Can you work these out from the model? Positions are in its coordinate system, mm. A direction names the side the tool comes from. Coordinates: 2 decimals unless noted, no trailing zeros. Loops run counter-clockwise (first coordinate to the right, second up) from the corner with the lowest first, then second, coordinate; pieces in that order, holes last.
```python
from build123d import *

# Parameters (mm, degrees)
SKETCH_W        = 16.8
SKETCH_H        = 16.8
SKETCH_R        = 2
PAD_DEPTH       = 16
SKETCH002_R     = 2
SKETCH002_R_2   = 3
PAD001_DEPTH    = 4
SKETCH003_W     = 12.4
SKETCH003_H     = 11.9
POCKET001_DEPTH = 12
SKETCH001_R     = 3.5
POCKET_DEPTH    = 4
POCKET002_DEPTH = 3.5
SKETCH005_R     = 2
POCKET003_DEPTH = 38.401
FILLET_R        = 2


with BuildPart() as part:
    # Sketch → Pad (new body)
    with BuildSketch(Plane.XY):
        Rectangle(SKETCH_W, SKETCH_H)
        Circle(SKETCH_R, mode=Mode.SUBTRACT)
    extrude(amount=PAD_DEPTH)

    # Sketch002 → Pad001 (join)
    with BuildSketch(Plane.XY.offset(16)):
        Polygon((-10, -10), (30, -10), (30, 10), (10, 10), (10, 30), (-10, 30), align=None)
        Circle(SKETCH002_R, mode=Mode.SUBTRACT)
        with Locations((0, 13.25)):
            Circle(SKETCH002_R_2, mode=Mode.SUBTRACT)
        with Locations((13.25, 0)):
            Circle(SKETCH002_R_2, mode=Mode.SUBTRACT)
    extrude(amount=PAD001_DEPTH)

    # Sketch003 → Pocket001 (cut)
    with BuildSketch(Plane.XY):
        with Locations((2.2, 2.45)):
            Rectangle(SKETCH003_W, SKETCH003_H)
    extrude(amount=POCKET001_DEPTH, mode=Mode.SUBTRACT)

    # Sketch001 (on Face5 of Pocket001) → Pocket (cut)
    with BuildSketch(Plane(origin=(0, 0, 16), x_dir=(1, 0, 0), z_dir=(0, 0, -1))):
        Circle(SKETCH001_R)
    extrude(amount=POCKET_DEPTH, mode=Mode.SUBTRACT)

    # Sketch004 (on Face7 of Pocket) → Pocket002 (cut)
    with BuildSketch(Plane(origin=(0, -3.5, 0), x_dir=(-1, 0, 0), z_dir=(0, 1, 0))):
        Polygon((4, 6), (2, 9.464102), (-2, 9.464102), (-4, 6), (-2, 2.535898), (2, 2.535898), align=None)
    extrude(amount=-POCKET002_DEPTH, mode=Mode.SUBTRACT)

    # Sketch005 (on Face1 of Pocket002) → Pocket003 (cut, through all)
    with BuildSketch(Plane.XZ.offset(8.4)):
        with Locations((0, 6)):
            Circle(SKETCH005_R)
    extrude(amount=-POCKET003_DEPTH, mode=Mode.SUBTRACT)

    # Fillet
    fillet_edges = [part.edges().sort_by_distance(p)[0] for p in [
        (-10, 30, 18),
        (10, 30, 18),
        (30, 10, 18),
        (30, -10, 18),
    ]]
    fillet(fillet_edges, radius=FILLET_R)


solid = part.part
```
Item 1: Suppose I cut it at A-A, the plane y = 13.25. Please give me the cut outline in (x, z).
Results are:
outline: (-10, 16) - (-3, 16) - (-3, 20) - (-10, 20) - close; (3, 16) - (10, 16) - (10, 20) - (3, 20) - close
Item 2: I need wall thicknesses on line 1 along Y through (x, z) = (0, 18.3); line 2 along Y through (x, z) = (13.25, 18.25); line 3 along X through (y, z) = (0, 15.15). Which ranges of each line are inside material? Lowest first, please.
Results are:
line 1: y = -10 to -2, 2 to 10.25, 16.25 to 30
line 2: y = -10 to -3, 3 to 10
line 3: x = -8.4 to -3.5, 3.5 to 8.4
Item 3: Suppose I cut it at D-D, the plane z = 5.25. Please give me the cut outline in (x, y).
Results are:
outline: (-8.4, -8.4) - (-1.85, -8.4) - (-1.85, -7) - (-3.57, -7) - (-3.57, -3.5) - (-4, -3.5) - (-4, 8.4) - (-8.4, 8.4) - close; (1.85, -8.4) - (8.4, -8.4) - (8.4, -3.5) - (3.57, -3.5) - (3.57, -7) - (1.85, -7) - close
Item 4: On a 3-axis mill with a long thin cutter (end or side, diameter ignored), from which of +Z, -Z, +X, -X, +Y, -Y can I reach the whole of each face in a straight line? I mean faces 1 (the face through (0, -8.4, 10)), 2 (the face through (-3.014, -5.226, 7.708)), 3 (the face through (19, 10, 18)), 4 (the face through (9, -10, 18)), 5 (the face through (-4, 8.4, 13)). Say none if no direction works.
Results are:
face 1: -Z, +X, -X, -Y
face 2: +Y
face 3: +Z, -Z, +X, +Y
face 4: +Z, -Z, +X, -X, -Y
face 5: -Z, +X, -X, +Y
Item 5: I'm going to push flat-ended pins straight in: P1, Ø6, axis at y = 21, z = 14, coming from the +X side; P2, Ø3.5, axis at x = 0.5, z = 7.5, coming from the +Y side; P3, Ø1, axis at y = -1, z = 5.5, coming from the +X side. Where does each tip first touch, or does it pass through?
Results are:
P1: stops at x = 10
P2: stops at y = -7
P3: stops at x = -4
Item 6: Suppose I cut it at C-C, the plane y = 0. Please give me the cut outline in (x, z).
Results are:
outline: (-10, 16) - (-8.4, 16) - (-8.4, 0) - (-4, 0) - (-4, 12) - (-3.5, 12) - (-3.5, 16) - (-2, 16) - (-2, 20) - (-10, 20) - close; (2, 16) - (3.5, 16) - (3.5, 12) - (8.4, 12) - (8.4, 16) - (10.25, 16) - (10.25, 20) - (2, 20) - close; (16.25, 16) - (30, 16) - (30, 20) - (16.25, 20) - close
Item 7: We'd pull the mould along Z, two halves only. Please class faces 6 (the face through (8.4, -4, 10)), 7 (the face through (5, 6, 20)), 8 (the face through (2, 2, 16)), 9 (the face through (0, -5, 9.464)): +Z half, -Z half, draft (parallel to the pull), parting line (faces both ways), or undercut.
Results are:
face 6: draft
face 7: +Z half
face 8: -Z half
face 9: undercut
